Could you check a few things on this model? Use its own coordinates, in mm. A direction names the side the tool comes from. Give positions to 0.01 mm unless a question says otherwise; leave off trailing zeros. Loops run counter-clockwise (first coordinate to the right, second up) from the corner with the lowest first, then second, coordinate; pieces in that order, holes last. Notation, with made-up numbers: (-29, 56.5) -> (15, 56.5) arc R16 cw to (15, 86.5) -> close; hole circle Ø10 at (31.5, -37). An arc over 180 degrees is marked (long way). Put each result on its own line as item: value.
```python
from build123d import *

# Parameters (mm, degrees)
EXTRUDE_1_DEPTH                 = 206
SKETCH_3_W                      = 252
SKETCH_3_H                      = 252
CUT_EXTRUDE_2_DEPTH             = 123.6
SKETCH_5_W                      = 210
SKETCH_5_H                      = 210
CUT_EXTRUDE_3_DEPTH             = 144.2
SHELL_1_T                       = -5
SKETCH_6_R                      = 50
CUT_EXTRUDE_4_DEPTH             = 455.80065963
RIB_START                       = -5
RIB_1_DEPTH                     = 10
PATTERN_CIRCULAR_2_COUNT        = 4
PATTERN_START                   = -5
PATTERN_CIRCULAR_2_COPY_1_DEPTH = 10
PATTERN_CIRCULAR_2_COPY_2_DEPTH = 10
PATTERN_CIRCULAR_2_COPY_3_DEPTH = 10


# Read off the part's stored shape, not the designer's step: the rib step
with BuildPart() as part:
    # Sketch 2 → Extrude 1 (new body)
    with BuildSketch(Plane.XY):
        Polygon((-183, 305), (-305, 183), (-305, -183), (-183, -305), (183, -305), (305, -183), (305, 183), (183, 305), align=None)
    extrude(amount=EXTRUDE_1_DEPTH)

    # Sketch 3 → Cut-Extrude 2 (cut)
    with BuildSketch(Plane.XY.offset(206)):
        Rectangle(SKETCH_3_W, SKETCH_3_H)
    extrude(amount=-CUT_EXTRUDE_2_DEPTH, mode=Mode.SUBTRACT)

    # Sketch 5 → Cut-Extrude 3 (cut)
    with BuildSketch(Plane.XY.offset(206)):
        Rectangle(SKETCH_5_W, SKETCH_5_H)
    extrude(amount=-CUT_EXTRUDE_3_DEPTH, mode=Mode.SUBTRACT)

    # Shell 1
    shell_1_openings = [part.faces().sort_by_distance(p)[0] for p in [
        (0, 0, 0),
    ]]
    offset(amount=SHELL_1_T, openings=shell_1_openings, kind=Kind.INTERSECTION)

    # Sketch 6 → Cut-Extrude 4 (cut, through all)
    with BuildSketch(Plane.XY.offset(61.8)):
        Circle(SKETCH_6_R)
    extrude(amount=-CUT_EXTRUDE_4_DEPTH, mode=Mode.SUBTRACT)

    # Rib 1 outline → Rib 1 (add)
    with BuildSketch(Plane(origin=(0, 91.5, 0), x_dir=(1, 0, 0), z_dir=(0, 1, 0)).offset(RIB_START)):
        Polygon((300, -112.109400071), (131, -82.310140331), (131, -201), (300, -201), align=None)
    rib_1 = extrude(amount=RIB_1_DEPTH)

    # Mirror 1: Rib 1 across plane
    add(rib_1.mirror(Plane.ZX))

    # Pattern Circular 2: Rib 1 ×4 about axis
    pattern_circular_2_axis = Axis((0, 0, 0), (0, 0, 1))
    for i in range(1, PATTERN_CIRCULAR_2_COUNT):
        add(rib_1.rotate(pattern_circular_2_axis, i * 360 / PATTERN_CIRCULAR_2_COUNT))

    # Pattern Circular 2 copy 1 sketch → Pattern Circular 2 copy 1 (add)
    with BuildSketch(Plane.YZ.offset(91.5).offset(PATTERN_START)):
        Polygon((300, 112.109400071), (131, 82.310140331), (131, 201), (300, 201), align=None)
    extrude(amount=PATTERN_CIRCULAR_2_COPY_1_DEPTH)

    # Pattern Circular 2 copy 2 sketch → Pattern Circular 2 copy 2 (add)
    with BuildSketch(Plane(origin=(0, 91.5, 0), x_dir=(-1, 0, 0), z_dir=(0, 1, 0)).offset(PATTERN_START)):
        Polygon((300, 112.109400071), (131, 82.310140331), (131, 201), (300, 201), align=None)
    extrude(amount=PATTERN_CIRCULAR_2_COPY_2_DEPTH)

    # Pattern Circular 2 copy 3 sketch → Pattern Circular 2 copy 3 (add)
    with BuildSketch(Plane(origin=(-91.5, 0, 0), x_dir=(0, -1, 0), z_dir=(-1, 0, 0)).offset(PATTERN_START)):
        Polygon((300, 112.109400071), (131, 82.310140331), (131, 201), (300, 201), align=None)
    extrude(amount=PATTERN_CIRCULAR_2_COPY_3_DEPTH)


solid = part.part
```
1. I'm going to push flat-ended pins straight in: pin 1 (2 mm diameter, centred on y = 222.5, z = 139, fed in from -X); pin 2 (1 mm diameter, centred on x = 226, z = 24.5, fed in from +Y). Where does each tip first touch, or does it pass through?
Recorded:
pin 1: stops at x = -266.5
pin 2: stops at y = 262.5
2. If we section it at B-B (x = 0): List the corners of the cut face in (y, z) for me, then the cut area to 3 significant figures.
Recorded:
outline: (-305, 0) -> (-300, 0) -> (-300, 201) -> (-131, 201) -> (-131, 77.4) -> (-110, 77.4) -> (-110, 56.8) -> (-50, 56.8) -> (-50, 61.8) -> (-105, 61.8) -> (-105, 82.4) -> (-126, 82.4) -> (-126, 206) -> (-305, 206) -> close; (50, 56.8) -> (110, 56.8) -> (110, 77.4) -> (131, 77.4) -> (131, 201) -> (300, 201) -> (300, 0) -> (305, 0) -> (305, 206) -> (126, 206) -> (126, 82.4) -> (105, 82.4) -> (105, 61.8) -> (50, 61.8) -> close
area: 6,000 mm^2
3. Thinking about a two-plate mould opening in Y: for faces 1 (the face through (-300, 3, 99)), 2 (the face through (-243, 245, 102)), 3 (the face through (174, 200, 201)), which applies, pulls with the +Y half, pulls with the -Y half, needs draft (parallel to the pull), parting line crosses it, or undercut?
Recorded:
face 1: undercut
face 2: pulls with the +Y half
face 3: undercut
4. If we section it at D-D (x = 197.5): List the corners of the cut face in (y, z) for me, then the cut area to 3 significant figures.
Recorded:
outline: (-290.5, 0) -> (-283.43, 0) -> (-283.43, 201) -> (-96.5, 201) -> (-96.5, 94.04) -> (-86.5, 94.04) -> (-86.5, 201) -> (86.5, 201) -> (86.5, 94.04) -> (96.5, 94.04) -> (96.5, 201) -> (283.43, 201) -> (283.43, 0) -> (290.5, 0) -> (290.5, 206) -> (-290.5, 206) -> close
area: 7,890 mm^2
5. If we section it at A-A (z = 41.5): List the corners of the cut face in (x, y) for me.
Recorded:
outline: (-305, -183) -> (-183, -305) -> (183, -305) -> (305, -183) -> (305, 183) -> (183, 305) -> (-183, 305) -> (-305, 183) -> close; hole (-300, -180.93) -> (-180.93, -300) -> (180.93, -300) -> (300, -180.93) -> (300, 180.93) -> (180.93, 300) -> (-180.93, 300) -> (-300, 180.93) -> close
6. For faces 4 (the face through (-48, 25, 61.8)), 5 (the face through (-86.5, 214, 154)), which set-ups out of +Z, -Z, +X, -X, +Y, -Y let a thin tool reach every point of the face, with its end or its side?
Recorded:
face 4: +Z
face 5: -Z
7. I need wall thicknesses on line 1 (Y direction, x = -50, z = 111.5); line 2 (Y direction, x = 0, z = 58.55). Which ranges of each line are inside material? Lowest first, please.
Recorded:
line 1: y = -305 to -300, -131 to -126, 126 to 131, 300 to 305
line 2: y = -305 to -300, -110 to -50, 50 to 110, 300 to 305
